from build123d import *

# Parameters (mm, degrees)
F1_DEPTH = 28.448
F2_DEPTH = 17.272
F3_DEPTH = 48.26
F0_W     = 18.288
F0_H     = 25.4
F4_DEPTH = 38.1
F5_R     = 6.35
F6_DEPTH = 53.34


with BuildPart() as f1:
    # F0 (on Top) → F1 (new body)
    with BuildSketch(Plane.XY):
        Polygon((41.672072, 25.770297), (-18.464064, 25.770297), (-18.464064, 20.690297), (-18.464064, -4.709703), (-18.464064, -9.789703), (41.672072, -9.789703), (53.163936, -3.154872), (53.163936, 19.135467), align=None)
    extrude(amount=F1_DEPTH)

    # F0 (on Top) → F2 (join)
    with BuildSketch(Plane.XY):
        Polygon((72.467936, 7.990297), (53.163936, 19.135467), (53.163936, -3.154872), align=None)
    extrude(amount=F2_DEPTH)

    # F0 (on Top) → F3 (join)
    with BuildSketch(Plane.XY):
        Polygon((-18.464064, 38.470297), (-46.912064, 38.470297), (-46.912064, 25.770297), (-36.752064, 25.770297), (-36.752064, 20.690297), (-18.464064, 20.690297), (-18.464064, 25.770297), align=None)
        Polygon((-18.464064, -9.789703), (-18.464064, -4.709703), (-36.752064, -4.709703), (-36.752064, -9.789703), (-46.912064, -9.789703), (-46.912064, -22.489703), (-18.464064, -22.489703), align=None)
    extrude(amount=F3_DEPTH)

    # F0 (on Top) → F4 (join)
    with BuildSketch(Plane.XY):
        with Locations((-27.608064, 7.990297)):
            Rectangle(F0_W, F0_H)
    extrude(amount=F4_DEPTH)

    # F5 (on face) → F6 (cut)
    with BuildSketch(Plane.XZ.offset(9.789703)):
        with Locations((16.587936, 14.224)):
            Circle(F5_R)
    extrude(amount=-F6_DEPTH, mode=Mode.SUBTRACT)


solid = f1.part
Can you work these out from the model? Positions are in its coordinate system, mm. A direction names the side the tool comes from. Round coordinates to 2 decimals unless told otherwise and drop trailing zeros. Order: outer loops, then holes, each group sorted by start corner. A loop starts at its lowest first (then second) coordinate and runs counter-clockwise, first axis right, second up. Notation, with made-up numbers: (24.25, 17) - (70.25, 17) arc R12 ccw to (70.25, 37) - close; hole circle Ø4 at (82.5, -9.75). An arc over 180 degrees is marked (long way). Answer in a Markdown table with one row per item.
(1) Suppose I cut it at D-D, the plane z = 13. Please give me the cut outline in (x, y).
From the geometry:
| item | result |
|---|---|
| outline | (-46.91, -22.49) - (-18.46, -22.49) - (-18.46, -9.79) - (10.36, -9.79) - (10.36, 25.77) - (-18.46, 25.77) - (-18.46, 38.47) - (-46.91, 38.47) - (-46.91, 25.77) - (-36.75, 25.77) - (-36.75, -9.79) - (-46.91, -9.79) - close; (22.82, -9.79) - (41.67, -9.79) - (72.47, 7.99) - (41.67, 25.77) - (22.82, 25.77) - close |
(2) Suppose I cut it at C-C, the plane x = -33.5. Please give me the cut outline in (y, z).
From the geometry:
| item | result |
|---|---|
| outline | (-22.49, 0) - (38.47, 0) - (38.47, 48.26) - (20.69, 48.26) - (20.69, 38.1) - (-4.71, 38.1) - (-4.71, 48.26) - (-22.49, 48.26) - close |
(3) If we mould it in two halves opening along Y, with no side actions, what happens to faces 6 (the face through (-1, 8, 0)), 7 (the face through (-28, 20.69, 43)), 8 (the face through (-33, -22.49, 24))? For each: released by +Y, released by -Y, zero draft, split by the parting line, or undercut.
From the geometry:
| item | result |
|---|---|
| face 6 | zero draft |
| face 7 | undercut |
| face 8 | released by -Y |
(4) Please list where these lines run through material, in increasing order: L1, parallel to Z at x = 16.5, y = 25; L2, parallel to X at y = 5.5, z = 26; L3, parallel to Z at x = 57, y = 10.5. Write a range as from..to.
From the geometry:
| item | result |
|---|---|
| L1 | z = 0..7.87, 20.57..28.45 |
| L2 | x = -36.75..53.16 |
| L3 | z = 0..17.27 |
(5) Suppose I cut it at A-A, the plane z = 40. Please give me the cut outline in (x, y).
From the geometry:
| item | result |
|---|---|
| outline | (-46.91, -22.49) - (-18.46, -22.49) - (-18.46, -4.71) - (-36.75, -4.71) - (-36.75, -9.79) - (-46.91, -9.79) - close; (-46.91, 25.77) - (-36.75, 25.77) - (-36.75, 20.69) - (-18.46, 20.69) - (-18.46, 38.47) - (-46.91, 38.47) - close |
(6) For P1, Ø5, axis at x = 20, y = -3.5, coming from the +Z side; P2, Ø10.5, axis at y = 9, z = 13.5, coming from the -X side; P3, Ø14, axis at x = 18, z = 11.5, coming from the -Y side, each with a flat end and sliding along its axis, tell me the tip position at first contact or that it passes through.
From the geometry:
| item | result |
|---|---|
| P1 | stops at z = 28.45 |
| P2 | stops at x = -36.75 |
| P3 | stops at y = -9.79 |
(7) Suppose I cut it at B-B, the plane y = 22. Please give me the cut outline in (x, z), plus the area to 3 significant figures.
From the geometry:
| item | result |
|---|---|
| outline | (-36.75, 0) - (48.2, 0) - (48.2, 28.45) - (-18.46, 28.45) - (-18.46, 48.26) - (-36.75, 48.26) - close; hole circle Ø12.7 at (16.59, 14.22) |
| area | 2,650 mm2 |
(8) Which directions (+Z, -Z, +X, -X, +Y, -Y) give clear straight access to the entire face, cutting with the end or side of a thin tool? Please do faces 1 (the face through (12, 25.77, 20)), 2 (the face through (17, 8, 28.448)), 3 (the face through (-46.912, -16, 24)), 4 (the face through (-27, -4.71, 43)), 5 (the face through (-36.752, 8, 18)).
From the geometry:
| item | result |
|---|---|
| face 1 | +Z, -Z, +X, +Y |
| face 2 | +Z, +X, +Y, -Y |
| face 3 | +Z, -Z, -X, +Y, -Y |
| face 4 | +Z, +X, -X |
| face 5 | +Z, -Z, -X |
